Verification items for the finished model (mm, model axes). Face numbers are marked on the shaded views. A direction names the side the tool comes from. Give positions to 0.01 mm unless a question says otherwise; leave off trailing zeros. Write each loop counter-clockwise with the first axis right and the second up, starting at its lowest first coordinate (ties: lowest second). Pieces come first, ordered by that corner, then holes. Notation, with made-up numbers: (-19.5, 26) -> (10.5, 26) arc R23 cw to (10.5, 49) -> close; hole circle Ø11 at (19, 78). An arc over 180 degrees is marked (long way). Answer as CSV lines item,"result".
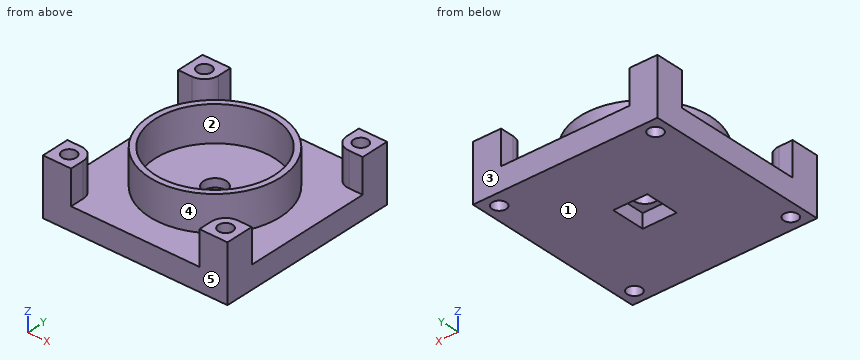
```python
from build123d import *

# Parameters (mm, degrees)
CROQUIS1_R              = 23
CROQUIS1_R_2            = 21
SALIENTE_EXTRUIR1_DEPTH = 12.5
CROQUIS2_W              = 65
CROQUIS2_H              = 65
CROQUIS2_R              = 2.5
SALIENTE_EXTRUIR2_DEPTH = 8
CROQUIS3_W              = 12
CROQUIS3_H              = 12
CORTAR_EXTRUIR1_DEPTH   = 5
CORTAR_EXTRUIR2_REACH   = 50.505
CROQUIS4_R              = 4
SALIENTE_EXTRUIR3_START = 12
CROQUIS5_R              = 2.5
SALIENTE_EXTRUIR3_DEPTH = 12


with BuildPart() as part:
    # Croquis1 → Saliente-Extruir1 (new body)
    with BuildSketch(Plane.XY):
        Circle(CROQUIS1_R)
        Circle(CROQUIS1_R_2, mode=Mode.SUBTRACT)
    extrude(amount=SALIENTE_EXTRUIR1_DEPTH)

    # Croquis2 → Saliente-Extruir2 (add)
    with BuildSketch(Plane.XY):
        Rectangle(CROQUIS2_W, CROQUIS2_H)
        with Locations((-27.550252532, 27.550252532)):
            Circle(CROQUIS2_R, mode=Mode.SUBTRACT)
        with Locations((27.550252532, 27.550252532)):
            Circle(CROQUIS2_R, mode=Mode.SUBTRACT)
        with Locations((-27.550252532, -27.550252532)):
            Circle(CROQUIS2_R, mode=Mode.SUBTRACT)
        with Locations((27.550252532, -27.550252532)):
            Circle(CROQUIS2_R, mode=Mode.SUBTRACT)
    extrude(amount=-SALIENTE_EXTRUIR2_DEPTH)

    # Croquis3 → Cortar-Extruir1 (cut)
    with BuildSketch(Plane(origin=(0, 0, -8), x_dir=(-1, 0, 0), z_dir=(0, 0, -1))):
        Rectangle(CROQUIS3_W, CROQUIS3_H)
    extrude(amount=-CORTAR_EXTRUIR1_DEPTH, mode=Mode.SUBTRACT)

    # Croquis4 → Cortar-Extruir2 (cut, up to next)
    with BuildSketch(Plane(origin=(0, 0, -3), x_dir=(-1, 0, 0), z_dir=(0, 0, -1)), mode=Mode.PRIVATE) as cortar_extruir2_sk1:
        Circle(CROQUIS4_R)
    cortar_extruir2_tool1 = extrude(cortar_extruir2_sk1.sketch, amount=-CORTAR_EXTRUIR2_REACH, mode=Mode.PRIVATE) & part.part
    add(cortar_extruir2_tool1.solids().sort_by_distance((0, 0, -3))[0], mode=Mode.SUBTRACT)

    # Croquis5 → Saliente-Extruir3 (add)
    # profile 1 of 4: a face of its own
    with BuildSketch(Plane.XY.offset(SALIENTE_EXTRUIR3_START)):
        with BuildLine():
            Line((27.600505063, 22.600505063), (32.5, 22.600505063))
            Line((32.5, 22.600505063), (32.5, 32.5))
            Line((32.5, 32.5), (22.600505063, 32.5))
            Line((22.600505063, 32.5), (22.600505063, 27.600505063))
            ThreePointArc((22.600505063, 27.600505063), (24.064971157, 24.064971157), (27.600505063, 22.600505063))
        make_face()
        with Locations((27.550252532, 27.550252532)):
            Circle(CROQUIS5_R, mode=Mode.SUBTRACT)
    # profile 2 of 4: a face of its own
    with BuildSketch(Plane.XY.offset(SALIENTE_EXTRUIR3_START)):
        with BuildLine():
            Line((-27.600505063, 22.600505063), (-32.5, 22.600505063))
            Line((-32.5, 22.600505063), (-32.5, 32.5))
            Line((-32.5, 32.5), (-22.600505063, 32.5))
            Line((-22.600505063, 32.5), (-22.600505063, 27.600505063))
            ThreePointArc((-22.600505063, 27.600505063), (-24.064971157, 24.064971157), (-27.600505063, 22.600505063))
        make_face()
        with Locations((-27.550252532, 27.550252532)):
            Circle(CROQUIS5_R, mode=Mode.SUBTRACT)
    # profile 3 of 4: a face of its own
    with BuildSketch(Plane.XY.offset(SALIENTE_EXTRUIR3_START)):
        with BuildLine():
            Line((-27.600505063, -22.600505063), (-32.5, -22.600505063))
            Line((-32.5, -22.600505063), (-32.5, -32.5))
            Line((-32.5, -32.5), (-22.600505063, -32.5))
            Line((-22.600505063, -32.5), (-22.600505063, -27.600505063))
            ThreePointArc((-22.600505063, -27.600505063), (-24.064971157, -24.064971157), (-27.600505063, -22.600505063))
        make_face()
        with Locations((-27.550252532, -27.550252532)):
            Circle(CROQUIS5_R, mode=Mode.SUBTRACT)
    # profile 4 of 4: a face of its own
    with BuildSketch(Plane.XY.offset(SALIENTE_EXTRUIR3_START)):
        with BuildLine():
            Line((27.600505063, -22.600505063), (32.5, -22.600505063))
            Line((32.5, -22.600505063), (32.5, -32.5))
            Line((32.5, -32.5), (22.600505063, -32.5))
            Line((22.600505063, -32.5), (22.600505063, -27.600505063))
            ThreePointArc((22.600505063, -27.600505063), (24.064971157, -24.064971157), (27.600505063, -22.600505063))
        make_face()
        with Locations((27.550252532, -27.550252532)):
            Circle(CROQUIS5_R, mode=Mode.SUBTRACT)
    extrude(amount=-SALIENTE_EXTRUIR3_DEPTH)


solid = part.part
```
1) Depth check by flat-ended pin: pin 1 (3 mm diameter, centred on x = -1.5, z = 6, fed in from -Y); pin 2 (11 mm diameter, centred on x = 27, y = 27, fed in from +Z); pin 3 (1 mm diameter, centred on x = 10, z = 7, fed in from +Y). Enter the tip coordinate at first touch or a pass-through.
Reported:
pin 1,"y = -23"
pin 2,"z = 12"
pin 3,"y = 20.95"
2) Section check D-D (x = 11). Record the boundary of the cut face in (y, z), and give its area (3 significant figures).
Reported:
outline,"(-32.5, -8) -> (32.5, -8) -> (32.5, 0) -> (20.2, 0) -> (20.2, 12.5) -> (17.89, 12.5) -> (17.89, 0) -> (-17.89, 0) -> (-17.89, 12.5) -> (-20.2, 12.5) -> (-20.2, 0) -> (-32.5, 0) -> close"
area,"578 mm²"
3) Tool access check on the marked faces 4 and 5. Record the directions out of +Z, -Z, +X, -X, +Y, -Y that give a thin tool (end or side, any length) a straight path to the whole face; none if there is none.
Reported:
face 4,"+Z"
face 5,"+Z, -Z, +X, -X, -Y"
4) Draft check along Y on the marked faces 1, 2 and 3. Enter one of: +Y half, -Y half, draft (parallel to the pull), parting line (faces both ways), or undercut.
Reported:
face 1,"draft"
face 2,"undercut"
face 3,"+Y half"
5) Scan lines: line 1 along X through (y, z) = (-27.5, 5); line 2 along Y through (x, z) = (0.5, -5.5); line 3 along X through (y, z) = (28, -4.25). Record each from-to range of solid material in increasing order.
Reported:
line 1,"-32.5 to -30.05, -25.05 to -22.6, 22.6 to 25.05, 30.05 to 32.5"
line 2,"-32.5 to -6, 6 to 32.5"
line 3,"-32.5 to -30.01, -25.09 to 25.09, 30.01 to 32.5"
6) Section check C-C (z = 4). State how many separate pieces and enclosed holes the cut face has, and give its area (3 significant figures).
Reported:
separate pieces,"5"
enclosed holes,"5"
area,"568 mm²"
7) Section check A-A (y = 0). Record the boundary of the cut face in (x, z).
Reported:
outline,"(-32.5, -8) -> (-6, -8) -> (-6, -3) -> (-4, -3) -> (-4, 0) -> (-21, 0) -> (-21, 12.5) -> (-23, 12.5) -> (-23, 0) -> (-32.5, 0) -> close; (4, -3) -> (6, -3) -> (6, -8) -> (32.5, -8) -> (32.5, 0) -> (23, 0) -> (23, 12.5) -> (21, 12.5) -> (21, 0) -> (4, 0) -> close"
